Geometry: final body of the model. Coordinates: model frame, mm. A direction names the side the tool comes from. Coordinates: 2 decimals unless noted, no trailing zeros. Loops run counter-clockwise (first coordinate to the right, second up) from the corner with the lowest first, then second, coordinate; pieces in that order, holes last. Notation, with made-up numbers: (-11.75, -6.5) -> (17.25, -6.5) arc R30 ccw to (17.25, 32.5) -> close; hole circle Ø7 at (64.25, 43.5). An arc over 180 degrees is marked (long way). One line per item, written item: value. Start each with the question number.
from build123d import *

# Parameters (mm, degrees)
BASE_FLANGE1_DEPTH           = 75
SKETCH5_R                    = 1.3
CUT_EXTRUDE1_DEPTH           = 10
SKETCH6_W                    = 89
SKETCH6_H                    = 5
CUT_EXTRUDE2_DEPTH           = 35
SKETCH9_W                    = 78.34
SKETCH9_H                    = 2
BOSS_EXTRUDE1_DEPTH          = 3
EDGE_FLANGE1_STRIP_W         = 14.66
EDGE_FLANGE1_STRIP_H         = 2
EDGE_FLANGE1_STRIP_CUT_DEPTH = 78.34
EDGE_FLANGE1_DEPTH           = 78.34
FILLET1_R                    = 2
SKETCH13_W                   = 24.17
SKETCH13_H                   = 34
SKETCH13_H_2                 = 19
SKETCH13_H_3                 = 39.67
CUT_EXTRUDE3_DEPTH           = 10
FILLET2_R                    = 2
SKETCH14_R                   = 1.37
CUT_EXTRUDE4_DEPTH           = 10


# Sheet-metal steps are written as plain solids
with BuildPart() as part:
    # Sketch1 → Base-Flange1 (new, symmetric)
    with BuildSketch(Plane.XY):
        with BuildLine():
            Line((-42.5, 10), (-42.5, 3.33))
            ThreePointArc((-42.5, 3.33), (-41.524665581, 0.975334419), (-39.17, 0))
            Line((-39.17, 0), (39.17, 0))
            ThreePointArc((39.17, 0), (41.524665581, 0.975334419), (42.5, 3.33))
            Line((42.5, 3.33), (42.5, 10))
            Line((42.5, 10), (44.5, 10))
            Line((44.5, 10), (44.5, 3.33))
            ThreePointArc((44.5, 3.33), (42.938879144, -0.438879144), (39.17, -2))
            Line((39.17, -2), (-39.17, -2))
            ThreePointArc((-39.17, -2), (-42.938879144, -0.438879144), (-44.5, 3.33))
            Line((-44.5, 3.33), (-44.5, 10))
            Line((-44.5, 10), (-42.5, 10))
        make_face()
    extrude(amount=BASE_FLANGE1_DEPTH, both=True)

    # Sketch5 → Cut-Extrude1 (cut)
    with BuildSketch(Plane(origin=(0, 0, 0), x_dir=(-1, 0, 0), z_dir=(0, 1, 0))):
        with Locations(Location((0, -23, 0), (0, 0, 90))):
            Circle(SKETCH5_R)
        with Locations(Location((16, -23, 0), (0, 0, 90))):
            Circle(SKETCH5_R)
        with Locations(Location((16, 12, 0), (0, 0, 90))):
            Circle(SKETCH5_R)
        with Locations(Location((0, 12, 0), (0, 0, 90))):
            Circle(SKETCH5_R)
        with Locations(Location((-16, 12, 0), (0, 0, 90))):
            Circle(SKETCH5_R)
        with Locations(Location((-16, -23, 0), (0, 0, 90))):
            Circle(SKETCH5_R)
        with Locations(Location((11, 12, 0), (0, 0, 90))):
            Circle(SKETCH5_R)
        with Locations(Location((5, 12, 0), (0, 0, 90))):
            Circle(SKETCH5_R)
        with Locations(Location((-5, 12, 0), (0, 0, 90))):
            Circle(SKETCH5_R)
        with Locations(Location((-11, 12, 0), (0, 0, 90))):
            Circle(SKETCH5_R)
        with Locations(Location((11, -23, 0), (0, 0, 90))):
            Circle(SKETCH5_R)
        with Locations(Location((5, -23, 0), (0, 0, 90))):
            Circle(SKETCH5_R)
        with Locations(Location((-5, -23, 0), (0, 0, 90))):
            Circle(SKETCH5_R)
        with Locations(Location((-11, -23, 0), (0, 0, 90))):
            Circle(SKETCH5_R)
        with Locations(Location((21, 12, 0), (0, 0, 90))):
            Circle(SKETCH5_R)
        with Locations(Location((21, -23, 0), (0, 0, 90))):
            Circle(SKETCH5_R)
        with Locations(Location((-21, -23, 0), (0, 0, 90))):
            Circle(SKETCH5_R)
        with Locations(Location((-21, 12, 0), (0, 0, 90))):
            Circle(SKETCH5_R)
    extrude(amount=-CUT_EXTRUDE1_DEPTH, mode=Mode.SUBTRACT)

    # Sketch6 → Cut-Extrude2 (cut)
    with BuildSketch(Plane.XZ.offset(2)):
        with Locations((0, 72.5)):
            Rectangle(SKETCH6_W, SKETCH6_H)
    extrude(amount=-CUT_EXTRUDE2_DEPTH, mode=Mode.SUBTRACT)

    # Sketch9 → Boss-Extrude1 (add)
    with BuildSketch(Plane.XY.offset(70)):
        with Locations((0, -1)):
            Rectangle(SKETCH9_W, SKETCH9_H)
    extrude(amount=BOSS_EXTRUDE1_DEPTH)

    # Edge-Flange1 strip (across the edge) → Edge-Flange1 strip cut (cut)
    with BuildSketch(Plane(origin=(-39.17, 0, 73), x_dir=(0, 0, -1), z_dir=(1, 0, 0))):
        with Locations((-4, -1)):
            Rectangle(EDGE_FLANGE1_STRIP_W, EDGE_FLANGE1_STRIP_H)
    extrude(amount=EDGE_FLANGE1_STRIP_CUT_DEPTH, mode=Mode.SUBTRACT)

    # Edge-Flange1 section (across the edge) → Edge-Flange1 (add)
    with BuildSketch(Plane(origin=(-39.17, 0, 73), x_dir=(0, 0, -1), z_dir=(1, 0, 0))):
        with BuildLine():
            Line((-2, 3.33), (-2, 10))
            Line((-2, 10), (0, 10))
            Line((0, 10), (0, 3.33))
            ThreePointArc((0, 3.33), (0.975334419, 0.975334419), (3.33, 0))
            Line((3.33, 0), (3.33, -2))
            ThreePointArc((3.33, -2), (-0.438879144, -0.438879144), (-2, 3.33))
        make_face()
    extrude(amount=EDGE_FLANGE1_DEPTH)

    # Fillet1
    fillet1_edges = [part.edges().sort_by_distance(p)[0] for p in [
        (-43.5, 10, -75),
        (43.5, 10, -75),
        (43.5, 10, 70),
        (-43.5, 10, 70),
        (-39.17, 10, 74),
        (39.17, 10, 74),
    ]]
    fillet(fillet1_edges, radius=FILLET1_R)

    # Sketch13 → Cut-Extrude3 (cut)
    with BuildSketch(Plane(origin=(0, 0, 0), x_dir=(1, 0, 0), z_dir=(0, 1, 0))):
        with Locations((-17.085, 48)):
            Rectangle(SKETCH13_W, SKETCH13_H)
        with Locations((17.085, 48)):
            Rectangle(SKETCH13_W, SKETCH13_H)
        with Locations((-17.085, 5.5)):
            Rectangle(SKETCH13_W, SKETCH13_H_2)
        with Locations((17.085, 5.5)):
            Rectangle(SKETCH13_W, SKETCH13_H_2)
        with Locations((-17.085, -39.835)):
            Rectangle(SKETCH13_W, SKETCH13_H_3)
        with Locations((17.085, -39.835)):
            Rectangle(SKETCH13_W, SKETCH13_H_3)
    extrude(amount=-CUT_EXTRUDE3_DEPTH, mode=Mode.SUBTRACT)

    # Fillet2
    fillet2_edges = [part.edges().sort_by_distance(p)[0] for p in [
        (-29.17, -1, -31),
        (-29.17, -1, -65),
        (-5, -1, -65),
        (-5, -1, -31),
        (5, -1, -31),
        (5, -1, -65),
        (29.17, -1, -65),
        (29.17, -1, -31),
        (-29.17, -1, 4),
        (-29.17, -1, -15),
        (-5, -1, -15),
        (-5, -1, 4),
        (5, -1, 4),
        (5, -1, -15),
        (29.17, -1, -15),
        (29.17, -1, 4),
        (-29.17, -1, 59.67),
        (-29.17, -1, 20),
        (-5, -1, 20),
        (-5, -1, 59.67),
        (5, -1, 59.67),
        (5, -1, 20),
        (29.17, -1, 20),
        (29.17, -1, 59.67),
    ]]
    fillet(fillet2_edges, radius=FILLET2_R)

    # Sketch14 → Cut-Extrude4 (cut)
    with BuildSketch(Plane(origin=(0, 0, 0), x_dir=(1, 0, 0), z_dir=(0, 1, 0))):
        with Locations(Location((-35.5, 71, 0), (0, 0, 270))):
            Circle(SKETCH14_R)
        with Locations(Location((35.5, 71, 0), (0, 0, 270))):
            Circle(SKETCH14_R)
        with Locations(Location((35.5, -66, 0), (0, 0, 270))):
            Circle(SKETCH14_R)
        with Locations(Location((-35.5, -66, 0), (0, 0, 270))):
            Circle(SKETCH14_R)
    extrude(amount=-CUT_EXTRUDE4_DEPTH, mode=Mode.SUBTRACT)


solid = part.part
1. Set-up query: faces 4 (the face through (-1, 0, -4)), 5 (the face through (42.4, 1.8, 70)), 6 (the face through (42.5, 7, -1)). Return all of +Z, -Z, +X, -X, +Y, -Y with unobstructed straight access to the full face (end or side cutting, diameter ignored); none if empty.
2. Section A-A on z = 18. Return the cut outline in (x, y).
3. Pin query (flat end, axial travel): pin 1 Ø1.6 at (y, z) = (-1, -55) entering from -X; pin 2 Ø1 at (x, y) = (-12.5, -1) entering from +Z; pin 3 Ø3 at (x, z) = (-24, 21) entering from +Y. Return the tip coordinate at first contact, or that it passes through.
4. Line query: L1, parallel to X at y = 3.5, z = 35.5; L2, parallel to Z at x = 9, y = -0.75; L3, parallel to X at y = -1.3, z = 66. Output: solid intervals per line, ascending. Write a range as [from, to].
5. Draft query along Z for faces 1 (the face through (-42.5, 7, -1)), 2 (the face through (35.56, -0.99, 64.63)), 3 (the face through (-42.5, 1.8, 70)). Return one class per face: released by +Z, released by -Z, zero draft, split by the parting line, or undercut.
Checks:
1. face 4: -Z, +Y
1. face 5: +Z, +X, +Y, -Y
1. face 6: +Z, -Z, +Y
2. outline: (-44.5, 3.33) arc R5.33 ccw to (-39.17, -2) -> (39.17, -2) arc R5.33 ccw to (44.5, 3.33) -> (44.5, 10) -> (42.5, 10) -> (42.5, 3.33) arc R3.33 cw to (39.17, 0) -> (-39.17, 0) arc R3.33 cw to (-42.5, 3.33) -> (-42.5, 10) -> (-44.5, 10) -> close
3. pin 1: x = -43.16
3. pin 2: z = 73.38
3. pin 3: y = 0
4. L1: [-44.5, -42.5], [42.5, 44.5]
4. L2: [-75, -65], [-31, -15], [4, 20], [59.67, 73.1]
4. L3: [-41.81, -36.87], [-34.13, 34.13], [36.87, 41.81]
5. face 1: zero draft
5. face 2: undercut
5. face 3: released by +Z
